from build123d import *

# Parameters (mm, degrees)
BOSS_EXTRUDE1_DEPTH     = 192.405
CUT_EXTRUDE1_DEPTH      = 193.632479478
CUT_EXTRUDE1_DEPTH_BACK = 193.632479478
SKETCH2_R               = 2.4892


with BuildPart() as part:
    # Sketch1 → Boss-Extrude1 (new body)
    with BuildSketch(Plane.XY):
        with BuildLine():
            Line((-0.893039494, 6.816751826), (-5.456960506, 4.181770802))
            ThreePointArc((-5.456960506, 4.181770802), (-5.953924651, 3.4375), (-6.35, 2.634981025))
            Line((-6.35, 2.634981025), (-6.35, -2.634981025))
            ThreePointArc((-6.35, -2.634981025), (-5.953924651, -3.4375), (-5.456960506, -4.181770802))
            Line((-5.456960506, -4.181770802), (-0.893039494, -6.816751826))
            ThreePointArc((-0.893039494, -6.816751826), (0, -6.875), (0.893039494, -6.816751826))
            Line((0.893039494, -6.816751826), (5.456960506, -4.181770802))
            ThreePointArc((5.456960506, -4.181770802), (5.953924651, -3.4375), (6.35, -2.634981025))
            Line((6.35, -2.634981025), (6.35, 2.634981025))
            ThreePointArc((6.35, 2.634981025), (5.953924651, 3.4375), (5.456960506, 4.181770802))
            Line((5.456960506, 4.181770802), (0.893039494, 6.816751826))
            ThreePointArc((0.893039494, 6.816751826), (0, 6.875), (-0.893039494, 6.816751826))
        make_face()
    extrude(amount=BOSS_EXTRUDE1_DEPTH)

    # Sketch2 → Cut-Extrude1 (cut, two sides: drawn at the far end of the back side and taken through both)
    with BuildSketch(Plane(origin=(0, 0, 0), x_dir=(-1, 0, 0), z_dir=(0, 0, -1)).offset(-CUT_EXTRUDE1_DEPTH_BACK)):
        Circle(SKETCH2_R)
    extrude(amount=CUT_EXTRUDE1_DEPTH + CUT_EXTRUDE1_DEPTH_BACK, mode=Mode.SUBTRACT)


solid = part.part
The listing builds one solid part. Answer for the finished solid, in the listing's coordinates (mm). Coordinates: 2 decimals unless noted, no trailing zeros. Write each loop counter-clockwise with the first axis right and the second up, starting at its lowest first coordinate (ties: lowest second). Pieces come first, ordered by that corner, then holes. Notation, with made-up numbers: M 27,89 L 69,89 A34 cw 69,120 Z; hole C 63,75 d2. An arc over 180 degrees is marked long. Write each question's results on one line, items separated by ' | '.
Item 1: Given P1, Ø8, axis at y = 4.5, z = 90.5, coming from the -X side; P2, Ø4, axis at y = 5, z = 84, coming from the +X side; P3, Ø3, axis at x = -2.5, z = 80.5, coming from the -Y side (3 decimals); P4, Ø4, axis at x = -4, z = 160, coming from the +Y side, each flat-ended and moving along its own axis, determine where each tip first touches the part or whether it passes through.
Answer below:
P1: x = -6.35 | P2: x = 6.19 | P3: y = -6.755 | P4: y = 6.18
Item 2: The part is cut by section B-B on z = 163. Determine the outline of the cut face in (x, y) (3 decimals).
Answer below:
outline: M -6.35,-2.635 A6.875 ccw -5.457,-4.182 L -0.893,-6.817 A6.875 ccw 0.893,-6.817 L 5.457,-4.182 A6.875 ccw 6.35,-2.635 L 6.35,2.635 A6.875 ccw 5.457,4.182 L 0.893,6.817 A6.875 ccw -0.893,6.817 L -5.457,4.182 A6.875 ccw -6.35,2.635 Z; hole C 0,0 d4.978
Item 3: For a pull along Y with two mould halves and no side action, classify faces 1 (the face through (-2.374, 0.748, 97.549)), 2 (the face through (3.21, 5.48, 94.86)), 3 (the face through (3, 0, 192.405)), 4 (the face through (-3.21, -5.48, 94.86)) as released by +Y, released by -Y, zero draft, split by the parting line, or undercut.
Answer below:
face 1: undercut | face 2: released by +Y | face 3: zero draft | face 4: released by -Y
Item 4: The part is cut by section A-A on y = 0. Determine the outline of the cut face in (x, z) (3 decimals).
Answer below:
outline: M -6.35,0 L -2.489,0 L -2.489,192.405 L -6.35,192.405 Z; M 2.489,0 L 6.35,0 L 6.35,192.405 L 2.489,192.405 Z
Item 5: Consider probe 1 along X at (y, z) = (0, 76.5); probe 2 along Y at (x, z) = (0, 18) (3 decimals); probe 3 along Y at (x, z) = (-3.25, 71.5). Determine where each line is inside the solid, lowest interval first. Write a range as [from, to].
Answer below:
probe 1: [-6.35, -2.49], [2.49, 6.35] | probe 2: [-6.875, -2.489], [2.489, 6.875] | probe 3: [-5.46, 5.46]
